The listing builds one solid part. Answer for the finished solid, in the listing's coordinates (mm). Face numbers are marked on the shaded views. Round coordinates to 2 decimals unless told otherwise and drop trailing zeros. Loops run counter-clockwise (first coordinate to the right, second up) from the corner with the lowest first, then second, coordinate; pieces in that order, holes last. Notation, with made-up numbers: (-28, -28) - (20, -28) arc R20 ccw to (20, -12) - close; hole circle Ø2 at (-15, 75.25). An arc over 180 degrees is marked (long way). One line per item, written item: value.
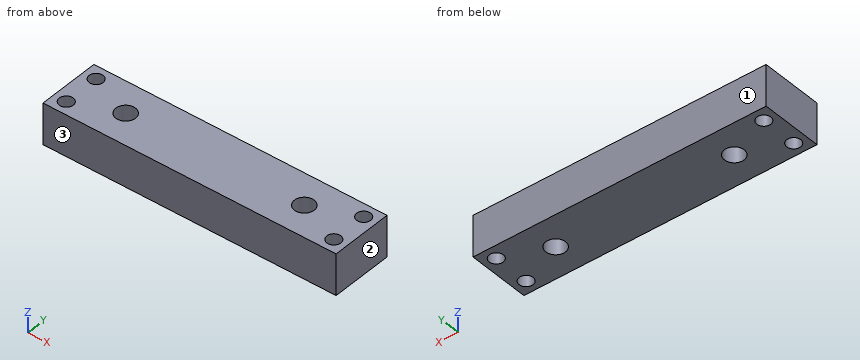
```python
from build123d import *

# Parameters (mm, degrees)
F0_W     = 356
F0_H     = 75
F0_R     = 8.5
F0_R_2   = 12
F0_R_3   = 13
F0_R_4   = 18
F1_DEPTH = 50
F2_D     = 24


with BuildPart() as f1:
    # F0 (on Top) → F1 (new body)
    with BuildSketch(Plane.XY):
        Rectangle(F0_W, F0_H)
        with Locations((-162.5, -22)):
            Circle(F0_R, mode=Mode.SUBTRACT)
        with Locations((162.5, -22)):
            Circle(F0_R_2, mode=Mode.SUBTRACT)
        with Locations((-108.5, 0)):
            Circle(F0_R_3, mode=Mode.SUBTRACT)
        with Locations((-162.5, 22)):
            Circle(F0_R, mode=Mode.SUBTRACT)
        with Locations((108.5, 0)):
            Circle(F0_R_4, mode=Mode.SUBTRACT)
        with Locations((162.5, 22)):
            Circle(F0_R, mode=Mode.SUBTRACT)
        with Locations((162.5, -22)):
            Circle(F0_R_2)
        with Locations((162.5, -22)):
            Circle(F0_R, mode=Mode.SUBTRACT)
        with Locations((108.5, 0)):
            Circle(F0_R_4)
        with Locations((108.5, 0)):
            Circle(F0_R_3, mode=Mode.SUBTRACT)
        with Locations((-108.5, 0)):
            Circle(F0_R_3)
        with Locations((108.5, 0)):
            Circle(F0_R_3)
    extrude(amount=F1_DEPTH)

    # F2 (through all)
    with Locations(Plane(origin=(0, 0, 0), x_dir=(1, 0, 0), z_dir=(0, 0, -1))):
        with Locations((-108.5, 0), (108.5, 0)):
            Hole(F2_D / 2)


solid = f1.part
```
1) A cutting plane is placed at C-C on x = 108.5. Give the vertices of the cut face in (y, z), and give its area (3 significant figures).
Final values:
outline: (-37.5, 0) - (-12, 0) - (-12, 50) - (-37.5, 50) - close; (12, 0) - (37.5, 0) - (37.5, 50) - (12, 50) - close
area: 2,550 mm2
2) A cutting plane is placed at B-B on z = 11. Give the vertices of the cut face in (x, y).
Final values:
outline: (-178, -37.5) - (178, -37.5) - (178, 37.5) - (-178, 37.5) - close; hole circle Ø17 at (-162.5, -22); hole circle Ø17 at (-162.5, 22); hole circle Ø24 at (-108.5, 0); hole circle Ø24 at (108.5, 0); hole circle Ø17 at (162.5, -22); hole circle Ø17 at (162.5, 22)
3) Consider L1, parallel to Y at x = 162.5, z = 27; L2, parallel to X at y = 22.5, z = 23; L3, parallel to X at y = 26.5, z = 30.5. Determine where each line is inside the solid, lowest interval first.
Final values:
L1: -37.5 to -30.5, -13.5 to 13.5, 30.5 to 37.5
L2: -178 to -170.99, -154.01 to 154.01, 170.99 to 178
L3: -178 to -169.71, -155.29 to 155.29, 169.71 to 178
4) A cutting plane is placed at A-A on y = -22. Give the vertices of the cut face in (x, z).
Final values:
outline: (-178, 0) - (-171, 0) - (-171, 50) - (-178, 50) - close; (-154, 0) - (154, 0) - (154, 50) - (-154, 50) - close; (171, 0) - (178, 0) - (178, 50) - (171, 50) - close
5) For a pull along Y with two mould halves and no side action, classify the marked faces 1, 2 and 3 as released by +Y, released by -Y, zero draft, split by the parting line, or undercut.
Final values:
face 1: released by +Y
face 2: zero draft
face 3: released by -Y
6) A cutting plane is placed at D-D on x = -162.5. Give the vertices of the cut face in (y, z).
Final values:
outline: (-37.5, 0) - (-30.5, 0) - (-30.5, 50) - (-37.5, 50) - close; (-13.5, 0) - (13.5, 0) - (13.5, 50) - (-13.5, 50) - close; (30.5, 0) - (37.5, 0) - (37.5, 50) - (30.5, 50) - close
